Study the drawing (mm; zero at the part's minimum x, y, z) and answer. A direction names the side the tool comes from. Round coordinates to 2 decimals unless told otherwise and drop trailing zeros. Order: outer loops, then holes, each group sorted by start corner. A loop starts at its lowest first (then second) coordinate and runs counter-clockwise, first axis right, second up. Notation, with made-up numbers: (17, 86.25) - (62, 86.25) arc R20 cw to (62, 117.25) - close; hole circle Ø4 at (61.5, 17). An arc over 180 degrees is marked (long way). Put each result on its own line as item: value.
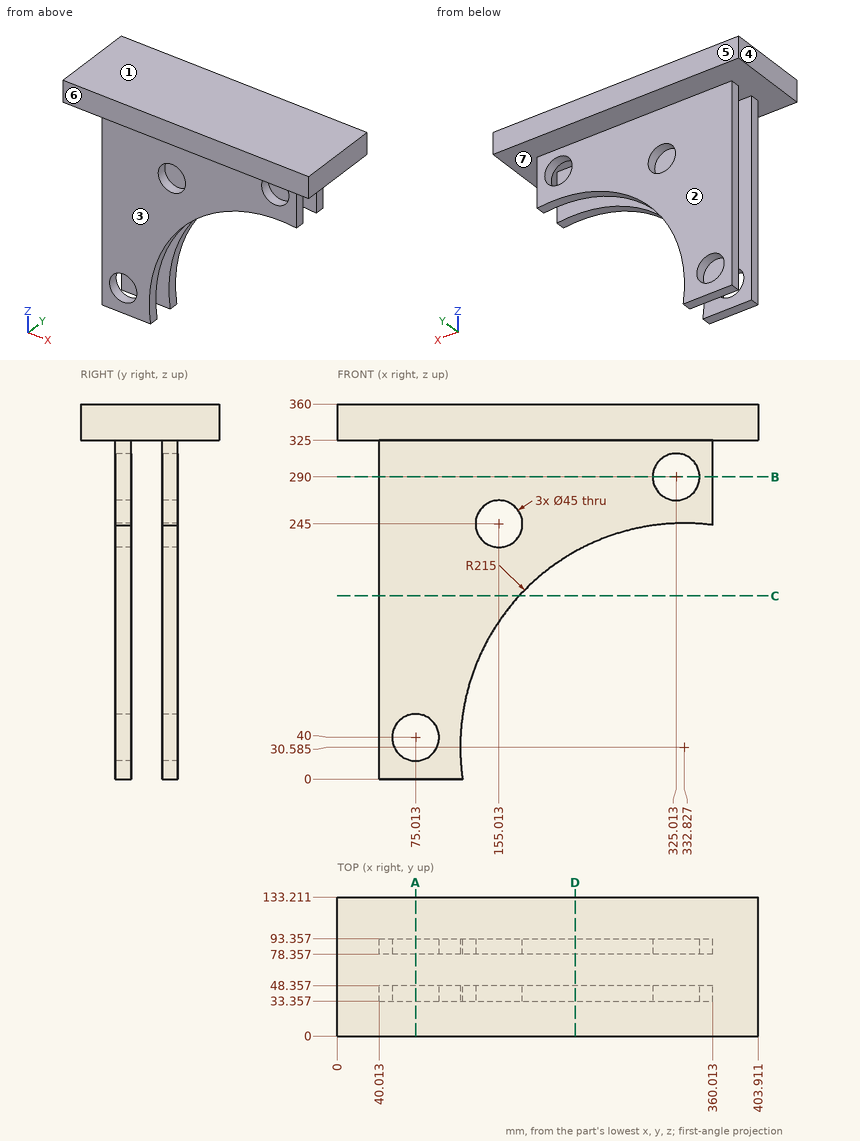
1) A cutting plane is placed at B-B on z = 290. Write down the section's boundary in (x, y), then the cut area to 3 significant figures.
Findings below:
outline: (40.01, 33.36) - (302.51, 33.36) - (302.51, 48.36) - (40.01, 48.36) - close; (40.01, 78.36) - (302.51, 78.36) - (302.51, 93.36) - (40.01, 93.36) - close; (347.51, 33.36) - (360.01, 33.36) - (360.01, 48.36) - (347.51, 48.36) - close; (347.51, 78.36) - (360.01, 78.36) - (360.01, 93.36) - (347.51, 93.36) - close
area: 8,250 mm2
2) Given pin 1 Ø1 at (x, y) = (114.5, 30.5) entering from -Z; pin 2 Ø2 at (x, z) = (342, 313.5) entering from -Y; pin 3 Ø4.5 at (y, z) = (40.5, 233) entering from -X, each flat-ended and moving along its own axis, determine where each tip first touches the part or whether it passes through.
Findings below:
pin 1: stops at z = 325
pin 2: stops at y = 33.36
pin 3: stops at x = 40.01
3) Straight lines are drawn through the part: L1, parallel to Y at x = 349, z = 281; L2, parallel to Z at x = 231.5, y = 94.5; L3, parallel to X at y = 38.5, z = 304 (1 decimal). For each, find the intervals that lie inside material, in ascending order. Write a range as from..to.
Findings below:
L1: y = 33.36..48.36, 78.36..93.36
L2: z = 325..360
L3: x = 40..307.4, 342.6..360
4) A cutting plane is placed at C-C on z = 176. Write down the section's boundary in (x, y), then the cut area to 3 significant figures.
Findings below:
outline: (40.01, 33.36) - (174.46, 33.36) - (174.46, 48.36) - (40.01, 48.36) - close; (40.01, 78.36) - (174.46, 78.36) - (174.46, 93.36) - (40.01, 93.36) - close
area: 4,030 mm2
5) For the marked faces 1, 2 and 3, determine the directions among +Z, -Z, +X, -X, +Y, -Y from which every point of the face is accessible in a straight line to the end or side of a thin tool.
Findings below:
face 1: +Z, +X, -X, +Y, -Y
face 2: -Z, +X, -X, +Y
face 3: -Z, +X, -X, -Y
6) For a pull along Y with two mould halves and no side action, classify the marked faces 4, 5, 6 and 7 as pulls with the +Y half, pulls with the -Y half, needs draft (parallel to the pull), parting line crosses it, or undercut.
Findings below:
face 4: needs draft
face 5: pulls with the +Y half
face 6: pulls with the -Y half
face 7: undercut
7) A cutting plane is placed at D-D on x = 228. Write down the section's boundary in (y, z), then the cut area to 3 significant figures.
Findings below:
outline: (0, 325) - (33.36, 325) - (33.36, 218.3) - (48.36, 218.3) - (48.36, 325) - (78.36, 325) - (78.36, 218.3) - (93.36, 218.3) - (93.36, 325) - (133.21, 325) - (133.21, 360) - (0, 360) - close
area: 7,860 mm2
8) A cutting plane is placed at A-A on x = 75. Write down the section's boundary in (y, z), then the cut area to 3 significant figures.
Findings below:
outline: (0, 325) - (33.36, 325) - (33.36, 62.5) - (48.36, 62.5) - (48.36, 325) - (78.36, 325) - (78.36, 62.5) - (93.36, 62.5) - (93.36, 325) - (133.21, 325) - (133.21, 360) - (0, 360) - close; (33.36, 0) - (48.36, 0) - (48.36, 17.5) - (33.36, 17.5) - close; (78.36, 0) - (93.36, 0) - (93.36, 17.5) - (78.36, 17.5) - close
area: 13,100 mm2
